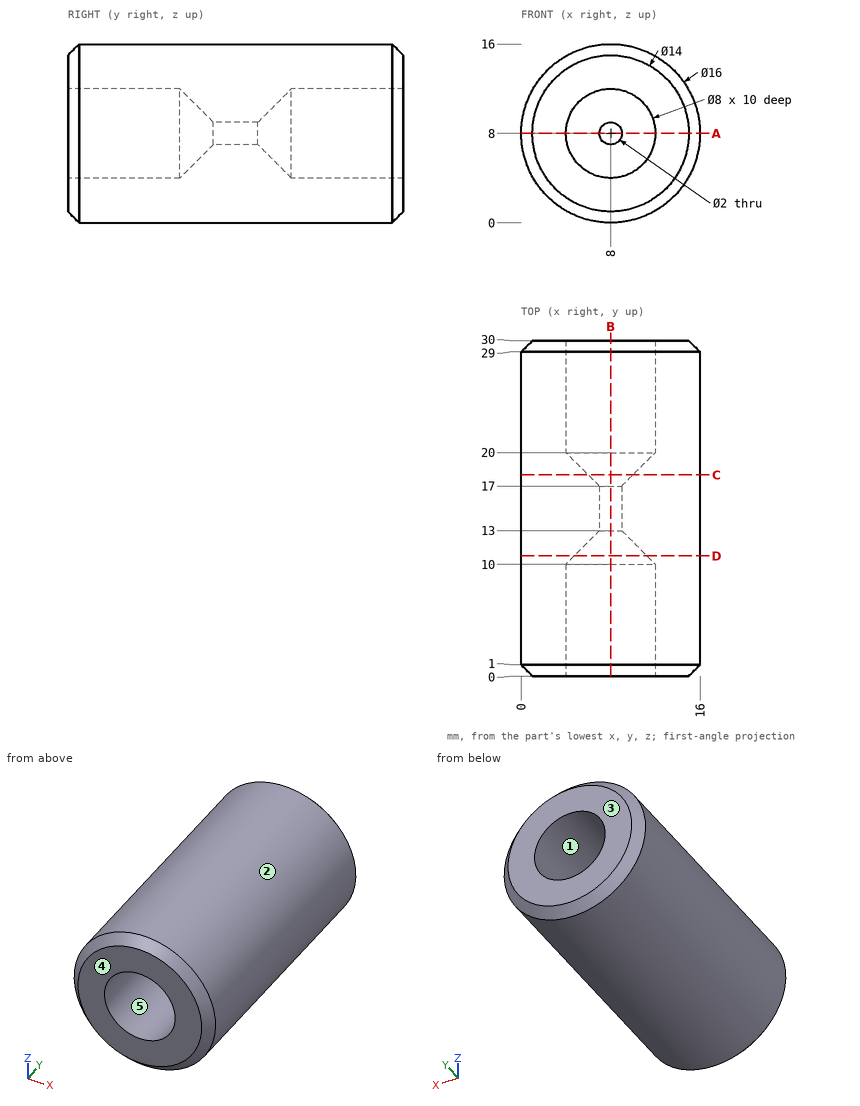
Geometry check sheet. Reference: drawing and pictorial views, mm from the part's lowest x, y, z. A direction names the side the tool comes from. Coordinates: 2 decimals unless noted, no trailing zeros. Order: outer loops, then holes, each group sorted by start corner. A loop starts at its lowest first (then second) coordinate and runs counter-clockwise, first axis right, second up.
Item 1: Section check A-A (z = 8). Enter the section's corners in (x, y).
Item 2: Depth check by flat-ended pin: pin 1 (3 mm diameter, centred on x = 4, z = 12.5, fed in from -Y); pin 2 (1 mm diameter, centred on y = 17.5, z = 9, fed in from +X); pin 3 (5 mm diameter, centred on x = 9, z = 7, fed in from -Y); pin 4 (3 mm diameter, centred on x = 8, z = 8, fed in from -Y). Enter the tip coordinate at first touch or a pass-through.
Item 3: Tool access check on the marked faces 4 and 5. Record the directions out of +Z, -Z, +X, -X, +Y, -Y that give a thin tool (end or side, any length) a straight path to the whole face; none if there is none.
Item 4: Section check B-B (x = 8). Enter the section's corners in (y, z).
Item 5: Section check C-C (y = 18). Enter the section's corners in (x, z), plus the area to 3 significant figures.
Item 6: Mould release check, pull along X, two halves, no side actions. Record for the marked faces 1, 2 and 3: released by +X, released by -X, zero draft, split by the parting line, or undercut.
Item 7: Scan lines: line 1 along X through (y, z) = (7.5, 8); line 2 along Z through (x, y) = (8, 15.45); line 3 along X through (y, z) = (15.75, 7.5). Record each from-to range of solid material in increasing order.
Item 8: Section check D-D (y = 10.75). Enter the section's corners in (x, z).
Check sheet entries:
1. outline: (0, 1) - (1, 0) - (4, 0) - (4, 10) - (7, 13) - (7, 17) - (4, 20) - (4, 30) - (1, 30) - (0, 29) - close; (9, 13) - (12, 10) - (12, 0) - (15, 0) - (16, 1) - (16, 29) - (15, 30) - (12, 30) - (12, 20) - (9, 17) - close
2. pin 1: stops at y = 0
2. pin 2: stops at x = 15.98
2. pin 3: stops at y = 10.09
2. pin 4: stops at y = 12.5
3. face 4: +Z, -Z, +X, -X, -Y
3. face 5: -Y
4. outline: (0, 1) - (1, 0) - (29, 0) - (30, 1) - (30, 4) - (20, 4) - (17, 7) - (13, 7) - (10, 4) - (0, 4) - close; (0, 12) - (10, 12) - (13, 9) - (17, 9) - (20, 12) - (30, 12) - (30, 15) - (29, 16) - (1, 16) - (0, 15) - close
5. outline: circle Ø16 at (8, 8); hole circle Ø4 at (8, 8)
5. area: 188 mm2
6. face 1: undercut
6. face 2: split by the parting line
6. face 3: zero draft
7. line 1: x = 0 to 4, 12 to 16
7. line 2: z = 0 to 7, 9 to 16
7. line 3: x = 0.02 to 7.13, 8.87 to 15.98
8. outline: circle Ø16 at (8, 8); hole circle Ø6.5 at (8, 8)
